Build history of the part. All positions in model axes, mm. A direction names the side the tool comes from. Coordinates: 2 decimals unless noted, no trailing zeros. Loops run counter-clockwise (first coordinate to the right, second up) from the corner with the lowest first, then second, coordinate; pieces in that order, holes last.
(1) Tool access for faces 4 (the face through (-8, 0, -2)), 5 (the face through (-79.23, 8.504, -2.95)), 6 (the face through (-17, 4, 2)): list every direction of +Z, -Z, +X, -X, +Y, -Y with a clear straight run to the whole face (end or side of a thin tool).
(2) Slice it at C-C (x = -138). Give the cut face in (y, z), and give its area (3 significant figures).
(3) Wall check: L1, parallel to X at y = 7.25, z = 0; L2, parallel to X at y = 5, z = 0; L3, parallel to Y at x = -32, z = -4.25. Give the ranges that are in metal, low to high.
(4) Two-plate mould, pull along X, no slides. Class faces 1 (the face through (-25, 1, -1)), 2 (the face through (-138, 9, 0)), 3 (the face through (-15.739, 13.93, -5.526)): pulls with the +X half, pulls with the -X half, needs draft (parallel to the pull), parting line crosses it, or undercut.
(5) Flat gauge pins, fed straight in: P1, Ø6, axis at y = 5.5, z = 1, coming from the -X side; P2, Ø10, axis at x = -103.5, z = -2.5, coming from the -Y side; P3, Ø1.5, axis at x = -91.5, y = 3, coming from the -Z side; P4, Ø2.5, axis at x = -13.5, y = 3.5, coming from the +Z side. Where does each tip first touch, or does it go through?
(6) Slice it at B-B (z = -1.25). Give the cut face in (x, y).
(7) Slice it at D-D (y = 15). Give the cut face in (x, z).
(8) Slice it at A-A (y = 7). Give the cut face in (x, z), and give its area (3 significant figures).
from build123d import *

# Parameters (mm, degrees)
SKETCH1_R           = 9
BOSS_EXTRUDE1_DEPTH = 9
SKETCH2_R           = 3
CUT_EXTRUDE1_DEPTH  = 29.053520278
SKETCH3_R           = 4
BOSS_EXTRUDE2_DEPTH = 9
SKETCH4_R           = 3.852623496
BOSS_EXTRUDE3_DEPTH = 110
SKETCH5_R           = 2
BOSS_EXTRUDE4_DEPTH = 10


with BuildPart() as part:
    # Sketch1 → Boss-Extrude1 (new body)
    with BuildSketch(Plane(origin=(0, 0, 0), x_dir=(1, 0, 0), z_dir=(0, 1, 0))):
        with BuildLine():
            ThreePointArc((-8.774964387, -2), (-7.03562364, 5.61248608), (0, 9))
            Line((0, 9), (-25, 9))
            Line((-25, 9), (-25, -2))
            Line((-25, -2), (-8.774964387, -2))
        make_face()
        Circle(SKETCH1_R)
    extrude(amount=BOSS_EXTRUDE1_DEPTH)

    # Sketch2 → Cut-Extrude1 (cut, through all)
    with BuildSketch(Plane.XZ):
        with Locations(Location((0, 0, 0), (0, 0, 270))):
            Circle(SKETCH2_R)
    extrude(amount=-CUT_EXTRUDE1_DEPTH, mode=Mode.SUBTRACT)



with BuildPart() as body_2:
    # Sketch3 → Boss-Extrude2 (new body)
    with BuildSketch(Plane(origin=(0, 0, 0), x_dir=(1, 0, 0), z_dir=(0, 1, 0))):
        with Locations(Location((-138, 0, 0), (0, 0, 270))):
            Circle(SKETCH3_R)
    extrude(amount=BOSS_EXTRUDE2_DEPTH)


with BuildPart() as part_1:
    add(part.part)

    add(body_2.part)  # Boss-Extrude3 merges body 2
    # Sketch4 → Boss-Extrude3 (add)
    with BuildSketch(Plane.ZY.offset(25)):
        with Locations(Location((-3.784788574, 4.743284234, 0), (0, 0, 180))):
            Circle(SKETCH4_R)
    extrude(amount=BOSS_EXTRUDE3_DEPTH)

    # Sketch5 → Boss-Extrude4 (add)
    with BuildSketch(Plane(origin=(0, 9, 0), x_dir=(1, 0, 0), z_dir=(0, 1, 0))):
        with Locations(Location((-14.38749457, 7, 0), (0, 0, 90))):
            Circle(SKETCH5_R)
    extrude(amount=BOSS_EXTRUDE4_DEPTH)


solid = part_1.part
Response values:
1. face 4: +Z, -Z, +X, -X, -Y
1. face 5: none
1. face 6: +Z, +Y, -Y
2. outline: (0, -4) - (9, -4) - (9, 4) - (0, 4) - close
2. area: 72.0 mm2
3. L1: x = -142 to -134, -25 to -3, 3 to 9
3. L2: x = -142 to -3, 3 to 9
3. L3: y = 0.92 to 8.57
4. face 1: undercut
4. face 2: needs draft
4. face 3: parting line crosses it
5. P1: stops at x = -142
5. P2: stops at y = 0.89
5. P3: stops at z = -7.51
5. P4: stops at z = 2
6. outline: (-141.8, 0) - (-134.2, 0) - (-134.2, 1.84) - (-25, 1.84) - (-25, 0) - (-2.73, 0) - (-2.73, 9) - (-25, 9) - (-25, 7.64) - (-134.2, 7.64) - (-134.2, 9) - (-141.8, 9) - close; (2.73, 0) - (8.91, 0) - (8.91, 9) - (2.73, 9) - close
7. outline: circle Ø4 at (-14.39, -7)
8. outline: (-135, -6.91) - (-25, -6.91) - (-25, -9) - (0, -9) arc R9 ccw (long way) to (-8.77, 2) - (-25, 2) - (-25, -0.66) - (-134.06, -0.66) arc R4 ccw (long way) to (-135, -2.65) - close; hole circle Ø6 at (0, 0)
8. area: 1,160 mm2
